Part model, mm, in its own coordinate system. Coordinates: 2 decimals unless noted, no trailing zeros. Write each loop counter-clockwise with the first axis right and the second up, starting at its lowest first coordinate (ties: lowest second). Pieces come first, ordered by that corner, then holes. Notation, with made-up numbers: (-11, 63) -> (29, 63) arc R22 cw to (29, 99) -> close; hole circle Ø5 at (7.5, 67.5). An arc over 180 degrees is marked (long way). One line per question, with ' | ' between items. Start each with the question number.
Item 1: Pin check, flat tip, straight feed: pin 1 (1.5 mm diameter, centred on y = -172, z = 58, fed in from +X). Stop position of the tip, or through.
Item 2: Probe probe 1 along Y at (x, z) = (267, 54); probe 2 along Y at (x, z) = (19, 102); probe 3 along X at (y, z) = (-30.5, 73.5). List the from-to ranges inside material, lowest first. Write a range as [from, to].
Item 3: Saw through at A-A (y = -132.5). List the corners of the cut face in (x, z), and give its area (3 significant figures).
Item 4: Saw through at B-B (z = 12). List the corners of the cut face in (x, y), and give its area (3 significant figures).
from build123d import *

# Parameters (mm, degrees)
F0_W     = 300
F0_H     = 150
F1_DEPTH = 200
F3_R     = 33.79899
F4_R     = 25


with BuildPart() as f1:
    # F0 (on Front) → F1 (new body)
    with BuildSketch(Plane.XZ):
        with Locations((150, 75)):
            Rectangle(F0_W, F0_H)
    extrude(amount=F1_DEPTH)

    # F3
    f3_edges = [f1.edges().sort_by_distance(p)[0] for p in [
        (300, -100, 150),
        (300, -100, 0),
        (300, 0, 75),
        (300, -200, 75),
    ]]
    fillet(f3_edges, radius=F3_R)

    # F4
    f4_edges = [f1.edges().sort_by_distance(p)[0] for p in [
        (0, -100, 150),
        (0, -100, 0),
        (0, 0, 75),
        (0, -200, 75),
    ]]
    fillet(f4_edges, radius=F4_R)


solid = f1.part
From the geometry:
1) pin 1: x = 299.62
2) probe 1: [-199.99, -0.01] | probe 2: [-199.27, -0.73] | probe 3: [0, 299.84]
3) outline: (0, 25) arc R25 ccw to (25, 0) -> (266.2, 0) arc R33.8 ccw to (300, 33.8) -> (300, 116.2) arc R33.8 ccw to (266.2, 150) -> (25, 150) arc R25 ccw to (0, 125) -> close | area: 44,200 mm2
4) outline: (3.65, -188) arc R25 ccw to (25, -200) -> (266.2, -200) arc R33.8 ccw to (292.03, -188) -> (292.03, -12) arc R33.8 ccw to (266.2, 0) -> (25, 0) arc R25 ccw to (3.65, -12) -> close | area: 57,300 mm2
